Source: CAD feature listing. Evaluate the final solid. Frame: model axes, mm. Face numbers are marked on the shaded views. A direction names the side the tool comes from. Coordinates: 2 decimals unless noted, no trailing zeros. Order: outer loops, then holes, each group sorted by start corner. A loop starts at its lowest first (then second) coordinate and runs counter-clockwise, first axis right, second up. Notation, with made-up numbers: (15.25, -37.75) - (51.25, -37.75) arc R24 cw to (51.25, -8.75) - close; hole circle Ø6 at (-22.75, -32.75). An arc over 180 degrees is marked (long way). One line per question, with ' | ' between items. Start each with the question number.
(1) Section D-D (x = 2.5). Return the cut outline in (y, z).
(2) Access query for the marked faces 1, 2 and 3. Directions: +Z, -Z, +X, -X, +Y, -Y. A direction counts if a zero-diameter tool reaches every point of the face in a straight line with its end or side. Return the directions, or none.
(3) Section A-A (z = 10). Return the cut outline in (x, y), then the cut area to 3 significant figures.
(4) Section C-C (y = -4). Return the cut outline in (x, z), then the cut area to 3 significant figures.
(5) Section B-B (x = 94.5). Return the cut outline in (y, z).
(6) Contact query for flat-ended pins moving along their axis: P1, Ø7, axis at x = 73, y = -6, coming from the -Z side; P2, Ø10, axis at x = 4.5, y = -21.5, coming from the +Z side; P3, Ø1, axis at x = 52, z = 9, coming from the +Y side; P4, Ø1.5, axis at x = 2.5, y = -8.5, coming from the +Z side. Output: stop coordinate, or through.
(7) Draft query along X for the marked faces 4, 5, 6 and 7. Return one class per face: +X half, -X half, draft (parallel to the pull), parting line (faces both ways), or undercut.
(8) Line query: line 1 along Y through (x, z) = (-9.5, 12.25); line 2 along Y through (x, z) = (12, 13); line 3 along Z through (x, y) = (19.5, -3.5). Output: solid intervals per line, ascending.
from build123d import *

# Parameters (mm, degrees)
EXTRUDE_5_DEPTH      = 15
CUT_EXTRUDE_8_DEPTH  = 5.2
CUT_EXTRUDE_9_DEPTH  = 15
CUT_EXTRUDE_10_DEPTH = 3.4
CUT_EXTRUDE_START    = -3.4
CUT_EXTRUDE_11_DEPTH = 3.4


with BuildPart() as part:
    # 草图1 → 凸台-拉伸5 (new body)
    with BuildSketch(Plane.XY):
        with BuildLine():
            Line((0, 0), (99.654203795, 8.309011134))
            ThreePointArc((99.654203795, 8.309011134), (110.217015146, 0.643574044), (104.203277967, -10.939468499))
            Line((104.203277967, -10.939468499), (11.372685429, -48.121199083))
            ThreePointArc((11.372685429, -48.121199083), (-22.25252281, -30.663509172), (0, 0))
        make_face()
    extrude(amount=EXTRUDE_5_DEPTH)

    # 草图9 → 切除-拉伸8 (cut)
    with BuildSketch(Plane(origin=(0, 0, 0), x_dir=(-1, 0, 0), z_dir=(0, 0, -1))):
        Polygon((-68.085389778, -2.37029612), (-73.03044485, -1.631086857), (-74.4743179, -11.290099671), (-69.529262828, -12.029308935), align=None)
    extrude(amount=-CUT_EXTRUDE_8_DEPTH, mode=Mode.SUBTRACT)

    # 草图9<5> → 切除-拉伸9 (cut)
    with BuildSketch(Plane(origin=(0, 0, 0), x_dir=(-1, 0, 0), z_dir=(0, 0, -1))):
        Polygon((-96.092530155, 3.045150664), (-72.850771317, -0.429132874), (-74.698794475, -12.791770554), (-97.940553313, -9.317487016), align=None)
    extrude(amount=-CUT_EXTRUDE_9_DEPTH, mode=Mode.SUBTRACT)

    # 草图1<11> → 切除-拉伸10 (cut)
    with BuildSketch(Plane.XY):
        with BuildLine():
            Line((0, 0), (99.654203795, 8.309011134))
            ThreePointArc((99.654203795, 8.309011134), (110.217015146, 0.643574044), (104.203277967, -10.939468499))
            Line((104.203277967, -10.939468499), (11.372685429, -48.121199083))
            ThreePointArc((11.372685429, -48.121199083), (-22.25252281, -30.663509172), (0, 0))
        make_face()
        with BuildLine():
            Line((6.86492087, -17.396188185), (6.623748603, -10.329097007))
            ThreePointArc((6.623748603, -10.329097007), (3.006492414, -6.630818399), (-1.003160039, -9.899532856))
            Line((-1.003160039, -9.899532856), (-2.038566002, -16.909799595))
            Line((-2.038566002, -16.909799595), (-8.279432627, -13.585115317))
            ThreePointArc((-8.279432627, -13.585115317), (-13.290863946, -14.868611764), (-12.464900415, -19.975429877))
            Line((-12.464900415, -19.975429877), (-6.911534313, -24.377251114))
            Line((-6.911534313, -24.377251114), (-12.91122867, -28.119658014))
            ThreePointArc((-12.91122867, -28.119658014), (-14.305403801, -33.101433069), (-9.469787817, -34.939536725))
            Line((-9.469787817, -34.939536725), (-2.881015752, -32.331091223))
            Line((-2.881015752, -32.331091223), (-2.639843484, -39.398182401))
            ThreePointArc((-2.639843484, -39.398182401), (0.977412704, -43.096461009), (4.987065158, -39.827746552))
            Line((4.987065158, -39.827746552), (6.022471121, -32.817479812))
            Line((6.022471121, -32.817479812), (12.263337746, -36.142164091))
            ThreePointArc((12.263337746, -36.142164091), (17.274769065, -34.858667644), (16.448805534, -29.751849531))
            Line((16.448805534, -29.751849531), (10.895439432, -25.350028294))
            Line((10.895439432, -25.350028294), (16.895133789, -21.607621394))
            ThreePointArc((16.895133789, -21.607621394), (18.28930892, -16.625846339), (13.453692935, -14.787742683))
            Line((13.453692935, -14.787742683), (6.86492087, -17.396188185))
        make_face(mode=Mode.SUBTRACT)
    extrude(amount=CUT_EXTRUDE_10_DEPTH, mode=Mode.SUBTRACT)

    # 草图25 → 切除-拉伸11 (cut)
    with BuildSketch(Plane.XY.offset(15).offset(CUT_EXTRUDE_START)):
        with BuildLine():
            Line((-2.038566002, -16.909799595), (-8.279432627, -13.585115317))
            ThreePointArc((-8.279432627, -13.585115317), (-13.290863946, -14.868611764), (-12.464900415, -19.975429877))
            Line((-12.464900415, -19.975429877), (-6.911534313, -24.377251114))
            Line((-6.911534313, -24.377251114), (-12.91122867, -28.119658014))
            ThreePointArc((-12.91122867, -28.119658014), (-14.305403801, -33.101433069), (-9.469787817, -34.939536725))
            Line((-9.469787817, -34.939536725), (-2.881015752, -32.331091223))
            Line((-2.881015752, -32.331091223), (-2.639843484, -39.398182401))
            ThreePointArc((-2.639843484, -39.398182401), (0.977412704, -43.096461009), (4.987065158, -39.827746552))
            Line((4.987065158, -39.827746552), (6.022471121, -32.817479812))
            Line((6.022471121, -32.817479812), (12.263337746, -36.142164091))
            ThreePointArc((12.263337746, -36.142164091), (17.274769065, -34.858667644), (16.448805534, -29.751849531))
            Line((16.448805534, -29.751849531), (10.895439432, -25.350028294))
            Line((10.895439432, -25.350028294), (16.895133789, -21.607621394))
            ThreePointArc((16.895133789, -21.607621394), (18.28930892, -16.625846339), (13.453692935, -14.787742683))
            Line((13.453692935, -14.787742683), (6.86492087, -17.396188185))
            Line((6.86492087, -17.396188185), (6.623748603, -10.329097007))
            ThreePointArc((6.623748603, -10.329097007), (3.006492414, -6.630818399), (-1.003160039, -9.899532856))
            Line((-1.003160039, -9.899532856), (-2.038566002, -16.909799595))
        make_face()
    extrude(amount=CUT_EXTRUDE_11_DEPTH, mode=Mode.SUBTRACT)


solid = part.part
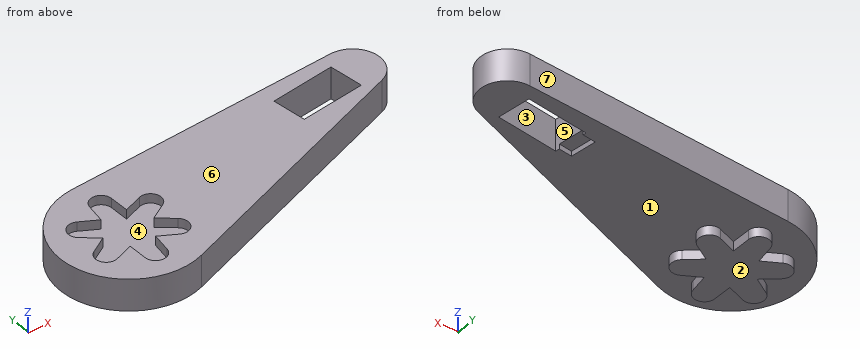
Response values:
1) outline: (-49.91, 3.4) - (-42.87, 3.4) - (-42.87, 0) - (-6.64, 0) - (-6.64, 3.4) - (0.21, 3.4) - (0.21, 15) - (-6.64, 15) - (-6.64, 11.6) - (-42.87, 11.6) - (-42.87, 15) - (-49.91, 15) - close
2) face 1: -Z | face 2: -Z, +X, -X, +Y, -Y | face 3: +Z, -Z
3) outline: (0, 0) arc R25 ccw (long way) to (11.37, -48.12) - (104.2, -10.94) arc R10 ccw to (99.65, 8.31) - close; hole (72.85, -0.43) - (74.7, -12.79) - (97.94, -9.32) - (96.09, 3.05) - close | area: 4,420 mm²
4) outline: (-11.62, 3.4) - (68.33, 3.4) - (68.33, 5.2) - (73.38, 5.2) - (73.38, 15) - (-11.62, 15) - close; (97.15, 3.4) - (110.21, 3.4) - (110.21, 15) - (97.15, 15) - close | area: 1,130 mm²
5) outline: (-14.83, 3.4) - (-9.83, 3.4) - (-9.83, 15) - (-14.83, 15) - close; (2.81, 3.4) - (7.88, 3.4) - (7.88, 15) - (2.81, 15) - close
6) P1: stops at z = 5.2 | P2: stops at z = 15 | P3: stops at y = 4.38 | P4: stops at z = 11.6
7) face 4: undercut | face 5: undercut | face 6: draft | face 7: -X half
8) line 1: y = -47.07 to -34.95, -25.99 to -22.33, -13.18 to -2.76 | line 2: y = -47.87 to -36, -26.23 to -24.66, -15.36 to 1 | line 3: z = 3.4 to 15
